Input: part model. Units: mm. Frame: model coordinates. Face numbers are marked on the shaded views. Round coordinates to 2 decimals unless told otherwise and drop trailing zeros. Order: outer loops, then holes, each group sorted by start corner. A loop starts at its lowest first (then second) coordinate and runs counter-clockwise, first axis right, second up. Notation, with made-up numbers: (70, 49) -> (120, 49) arc R20 cw to (120, 80) -> close; hole circle Ø3 at (20.5, 14.5). An arc over 180 degrees is marked (long way). Use a Markdown table: item, result.
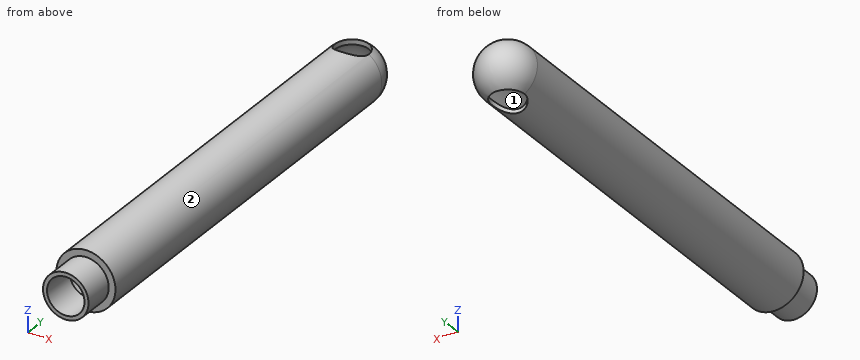
from build123d import *

# Parameters (mm, degrees)
CUT_EXTRUDE1_DEPTH      = 608.258594011
CUT_EXTRUDE1_DEPTH_BACK = 608.258594011
SKETCH2_R               = 21


with BuildPart() as part:
    # Sketch1 → Revolve1 (revolve)
    with BuildSketch(Plane.XY, mode=Mode.PRIVATE) as revolve1_sk:
        with BuildLine():
            Line((23.5, 0), (28.5, 0))
            Line((28.5, 0), (28.5, 40))
            Line((28.5, 40), (37, 40))
            Line((37, 40), (37, 568))
            ThreePointArc((37, 568), (26.162950904, 594.162950904), (0, 605))
            Line((0, 605), (0, 600))
            ThreePointArc((0, 600), (22.627416998, 590.627416998), (32, 568))
            Line((32, 568), (32, 45))
            Line((32, 45), (23.5, 45))
            Line((23.5, 45), (23.5, 0))
        make_face()
    revolve(revolve1_sk.sketch.rotate(Axis((0, 0, 0), (0, 1, 0)), 90), axis=Axis((0, 0, 0), (0, 1, 0)))

    # Sketch2 → Cut-Extrude1 (cut, two sides: drawn at the far end of the back side and taken through both)
    with BuildSketch(Plane.XY.offset(-CUT_EXTRUDE1_DEPTH_BACK)):
        with Locations((0, 568)):
            Circle(SKETCH2_R)
    extrude(amount=CUT_EXTRUDE1_DEPTH + CUT_EXTRUDE1_DEPTH_BACK, mode=Mode.SUBTRACT)


solid = part.part
1) Pull-direction query (Z, two-part tool) for the marked faces 1 and 2; classes: +Z half, -Z half, draft (parallel to the pull), parting line (faces both ways), or undercut.
Results found:
| item | result |
|---|---|
| face 1 | undercut |
| face 2 | parting line |
2) Cut plane B-B on z = 0. Return loops of the section in (x, y), and give its area (3 significant figures).
Results found:
| item | result |
|---|---|
| outline | (-37, 40) -> (-28.5, 40) -> (-28.5, 0) -> (-23.5, 0) -> (-23.5, 45) -> (-32, 45) -> (-32, 568) arc R32 cw to (32, 568) -> (32, 45) -> (23.5, 45) -> (23.5, 0) -> (28.5, 0) -> (28.5, 40) -> (37, 40) -> (37, 568) arc R37 ccw to (-37, 568) -> close |
| area | 6,310 mm² |
3) Pin query (flat end, axial travel): pin 1 Ø19 at (x, z) = (-15, -0.5) entering from +Y; pin 2 Ø3 at (x, y) = (9, 116.5) entering from +Z; pin 3 Ø2 at (y, z) = (163.5, 9) entering from +X. Return the tip coordinate at first contact, or that it passes through.
Results found:
| item | result |
|---|---|
| pin 1 | stops at y = 604.59 |
| pin 2 | stops at z = 36.23 |
| pin 3 | stops at x = 36.12 |
4) Cut plane C-C on y = 273.5. Return loops of the section in (x, z), and give its area (3 significant figures).
Results found:
| item | result |
|---|---|
| outline | circle Ø74 at (0, 0); hole circle Ø64 at (0, 0) |
| area | 1,080 mm² |
5) Line query: L1, parallel to X at y = 15.5, z = 0; L2, parallel to X at y = 305, z = 0; L3, parallel to Y at x = -1, z = -31. Output: solid intervals per line, ascending. Write a range as [from, to].
Results found:
| item | result |
|---|---|
| L1 | x = [-28.5, -23.5], [23.5, 28.5] |
| L2 | x = [-37, -32], [32, 37] |
| L3 | y = [40, 45] |
6) Cut plane A-A on x = 0. Return loops of the section in (y, z).
Results found:
| item | result |
|---|---|
| outline | (0, -28.5) -> (40, -28.5) -> (40, -37) -> (547, -37) -> (547, -32) -> (45, -32) -> (45, -23.5) -> (0, -23.5) -> close; (0, 23.5) -> (45, 23.5) -> (45, 32) -> (547, 32) -> (547, 37) -> (40, 37) -> (40, 28.5) -> (0, 28.5) -> close; (589, -30.46) arc R37 ccw to (589, 30.46) -> (589, 24.15) arc R32 cw to (589, -24.15) -> close |
